Geometry: final body of the model. Coordinates: model frame, mm. A direction names the side the tool comes from. Give positions to 0.01 mm unless a question says otherwise; leave off trailing zeros. Write each loop counter-clockwise with the first axis right and the second up, starting at its lowest first coordinate (ties: lowest second). Pieces come first, ordered by that corner, then holes. Notation, with made-up numbers: M 22,-27 L 51,-27 A10 cw 51,-20 Z; hole C 11,21.25 d3. An arc over 180 degrees is marked long. Use one line per item in the form item = value. Start each with the question number.
Item 1: Section query C-C on x = -5. Return loops of the section in (y, z), then the cut area to 3 significant figures.
Item 2: Contact query for flat-ended pins moving along their axis: P1, Ø2, axis at x = -9, z = -2, coming from the -Y side; P2, Ø2, axis at y = 1, z = 17, coming from the -X side; P3, Ø1, axis at x = 4, y = 20, coming from the -Z side; P4, Ø1.8, axis at x = 0, z = 19.5, coming from the -Y side. Output: stop coordinate, or through.
Item 3: Access query for faces 1 (the cylindrical face through (3.708, -0.616, -1.352)), 2 (the flat face through (0, 25.2, 0)), 3 (the flat face through (8, -8, 2)), 4 (the cylindrical face through (-0.1, 1, 23.5)), 5 (the cylindrical face through (-14.78, 6.08, 6.13)). Directions: +Z, -Z, +X, -X, +Y, -Y. A direction counts if a zero-diameter tool reaches every point of the face in a straight line with its end or side. Return the directions, or none.
Item 4: Pull-direction query (X, two-part tool) for faces 6 (the cylindrical face through (0, 1, -18)), 7 (the conical face through (7.7, -1.9, -0.1)), 8 (the cylindrical face through (-6.586, 19.678, -10.329)), 9 (the flat face through (4, 1, -17)); classes: released by +X, released by -X, zero draft, split by the parting line, or undercut.
Item 5: Section query B-B on y = 1. Return loops of the section in (x, z).
Item 6: Section query A-A on x = 0. Return loops of the section in (y, z), then the cut area to 3 significant figures.
Item 7: Section query D-D on z = 8. Return loops of the section in (x, y), then the cut area to 3 significant figures.
Item 8: Material intervals for line 1 along Z through (x, y) = (0, 1.05); line 2 along Y through (x, z) = (-1, -3.5); line 3 along X through (y, z) = (1, 19), sorted ascending. Write a range as from..to.
from build123d import *

# Parameters (mm, degrees)
HOLE_WIZARD_M4_1_D     = 3.3
HOLE_WIZARD_M4_1_DEPTH = 7.5
HOLE_WIZARD_M4_1_TIP   = 0.991420021
CUT_EXTRUDE_START      = 10.2
SKETCH_5_W             = 10.320177725
SKETCH_5_H             = 3.570001837
SKETCH_5_W_2           = 11.817937116
SKETCH_5_H_2           = 2.503104736
CUT_EXTRUDE_1_DEPTH    = 5
SKETCH_6_R             = 1.5
EXTRUDE_1_DEPTH        = 2
EXTRUDE_2_DEPTH        = 15


with BuildPart() as part:
    # 草图1 → 旋转1 (revolve)
    with BuildSketch(Plane.XY):
        Polygon((0, 0), (-16, 0), (-16, 12), (-13, 12), (-13, 14), (-12.25, 14), (-12.25, 25.2), (0, 25.2), align=None)
    revolve(axis=Axis((0, 25.2, 0), (0, -1, 0)))

    # 草图2 → 旋转2 (revolve)
    with BuildSketch(Plane.XY):
        Polygon((8, -10.2), (5.5, -10.2), (5.5, -2.7), (4, -2.7), (4, -1.25), (3.5, -1.25), (3.5, 0), (8, 0), align=None)
    revolve(axis=Axis((8, 0, 0), (0, -1, 0)))

    # M4 螺纹孔1
    with Locations(Plane(origin=(0, -10.2, 0), x_dir=(-1, 0, 0), z_dir=(0, -1, 0))):
        with Locations((-8, 0)):
            Hole(HOLE_WIZARD_M4_1_D / 2, depth=HOLE_WIZARD_M4_1_DEPTH)
            with Locations((0, 0, -(HOLE_WIZARD_M4_1_DEPTH + HOLE_WIZARD_M4_1_TIP / 2))):  # 118° drill point
                Cone(0, HOLE_WIZARD_M4_1_D / 2, HOLE_WIZARD_M4_1_TIP, mode=Mode.SUBTRACT)

    # 草图5 → 切除-拉伸1 (cut)
    with BuildSketch(Plane.XZ.offset(CUT_EXTRUDE_START)):
        with Locations((7.585780696, 3.785000919)):
            Rectangle(SKETCH_5_W, SKETCH_5_H)
        with Locations((6.836901, -3.251552368)):
            Rectangle(SKETCH_5_W_2, SKETCH_5_H_2)
    extrude(amount=-CUT_EXTRUDE_1_DEPTH, mode=Mode.SUBTRACT)

    # 草图6 → 凸台-拉伸1 (add)
    with BuildSketch(Plane.XZ):
        with BuildLine():
            Line((4, 19.5), (4, -19.5))
            ThreePointArc((4, -19.5), (0, -23.5), (-4, -19.5))
            Line((-4, -19.5), (-4, 19.5))
            ThreePointArc((-4, 19.5), (0, 23.5), (4, 19.5))
        make_face()
        with Locations((0, -19.5)):
            Circle(SKETCH_6_R, mode=Mode.SUBTRACT)
        with Locations((0, 19.5)):
            Circle(SKETCH_6_R, mode=Mode.SUBTRACT)
    extrude(amount=-EXTRUDE_1_DEPTH)

    # 草图7 → 凸台-拉伸2 (add)
    with BuildSketch(Plane(origin=(0, 0, 0), x_dir=(0, 0, -1), z_dir=(1, 0, 0))):
        with BuildLine():
            Line((-1.687384392, 24.513955372), (1.687384392, 24.513955372))
            ThreePointArc((1.687384392, 24.513955372), (2.169302813, 24.032036951), (1.687384392, 23.550118529))
            Line((1.687384392, 23.550118529), (-1.687384392, 23.550118529))
            ThreePointArc((-1.687384392, 23.550118529), (-2.169302813, 24.032036951), (-1.687384392, 24.513955372))
        make_face()
    extrude(amount=-EXTRUDE_2_DEPTH)


solid = part.part
Answer sheet:
q1.outline = M 0,-15.2 L 12,-15.2 L 12,-12 L 14,-12 L 14,-11.18 L 25.2,-11.18 L 25.2,11.18 L 14,11.18 L 14,12 L 12,12 L 12,15.2 L 0,15.2 Z
q1.area = 663 mm2
q2.P1 = 0
q2.P2 = -4
q2.P3 = -11.74
q2.P4 = through
q3.face_1 = -Y
q3.face_2 = +Z, -Z, +X, -X, +Y
q3.face_3 = +Z, +X, -X, -Y
q3.face_4 = +Z, +Y, -Y
q3.face_5 = +Y
q4.face_6 = undercut
q4.face_7 = undercut
q4.face_8 = split by the parting line
q4.face_9 = released by +X
q5.outline = M -4,-19.5 A4 ccw 4,-19.5 L 4,-15.49 A16 ccw 4,15.49 L 4,19.5 A4 ccw -4,19.5 L -4,15.49 A16 ccw -4,-15.49 Z; hole C 0,-19.5 d3; hole C 0,19.5 d3
q6.outline = M 0,-23.5 L 2,-23.5 L 2,-21 L 0,-21 Z; M 0,-18 L 2,-18 L 2,-16 L 12,-16 L 12,-13 L 14,-13 L 14,-12.25 L 25.2,-12.25 L 25.2,12.25 L 14,12.25 L 14,13 L 12,13 L 12,16 L 2,16 L 2,18 L 0,18 Z; M 0,21 L 2,21 L 2,23.5 L 0,23.5 Z
q6.area = 728 mm2
q7.outline = M -13.86,0 L 13.86,0 L 13.86,12 L 10.25,12 L 10.25,14 L 9.28,14 L 9.28,25.2 L -9.28,25.2 L -9.28,14 L -10.25,14 L -10.25,12 L -13.86,12 Z
q7.area = 581 mm2
q8.line_1 = -23.5..-21, -18..18, 21..23.5
q8.line_2 = 0..25.2
q8.line_3 = -4..-1.41, 1.41..4
